from build123d import *

# Parameters (mm, degrees)
SKETCH1_R           = 30
BOSS_EXTRUDE1_DEPTH = 21.25
CUT_EXTRUDE1_DEPTH  = 5
SKETCH5_R           = 1.8
CUT_EXTRUDE2_DEPTH  = 48.45063224
CUT_EXTRUDE3_DEPTH  = 13
SKETCH10_W          = 15
SKETCH10_H          = 9.25
CUT_EXTRUDE6_DEPTH  = 28
FILLET6_R           = 5
FILLET7_R           = 5


with BuildPart() as part:
    # Sketch1 → Boss-Extrude1 (new body)
    with BuildSketch(Plane.XY):
        Circle(SKETCH1_R)
    extrude(amount=BOSS_EXTRUDE1_DEPTH)

    # Sketch2 → Cut-Extrude1 (cut)
    with BuildSketch(Plane.XY.offset(21.25)):
        Polygon((0, 7.361215932), (-6.375, 3.680607966), (-6.375, -3.680607966), (0, -7.361215932), (6.375, -3.680607966), (6.375, 3.680607966), align=None)
    extrude(amount=-CUT_EXTRUDE1_DEPTH, mode=Mode.SUBTRACT)

    # Sketch4 → Cut-Revolve1 (revolve, cut)
    with BuildSketch(Plane(origin=(0, 0, 0), x_dir=(1, 0, 0), z_dir=(0, 1, 0)), mode=Mode.PRIVATE) as cut_revolve1_sk:
        Polygon((30, -19.25), (26, -15.25), (26, -6), (30, -2), align=None)
    revolve(cut_revolve1_sk.sketch.rotate(Axis((0, 0, -12.64061748), (0, 0, 1)), 180), axis=Axis((0, 0, -12.64061748), (0, 0, 1)), mode=Mode.SUBTRACT)

    # Sketch5 → Cut-Extrude2 (cut, through all)
    with BuildSketch(Plane.XY.offset(21.25)):
        with Locations((-17.320508076, -10)):
            Circle(SKETCH5_R)
        with Locations((17.320508076, -10)):
            Circle(SKETCH5_R)
        with Locations((0, 20)):
            Circle(SKETCH5_R)
    extrude(amount=-CUT_EXTRUDE2_DEPTH, mode=Mode.SUBTRACT)

    # Sketch6 → Cut-Extrude3 (cut)
    with BuildSketch(Plane(origin=(0, 0, 0), x_dir=(-1, 0, 0), z_dir=(0, 0, -1))):
        Polygon((7.361215932, 0), (3.680607966, 6.375), (-3.680607966, 6.375), (-7.361215932, 0), (-3.680607966, -6.375), (3.680607966, -6.375), align=None)
    extrude(amount=-CUT_EXTRUDE3_DEPTH, mode=Mode.SUBTRACT)

    # Sketch10 → Cut-Extrude6 (cut)
    with BuildSketch(Plane(origin=(0, 40, 0), x_dir=(1, 0, 0), z_dir=(0, 1, 0))):
        with Locations((0, -10.625)):
            Rectangle(SKETCH10_W, SKETCH10_H)
    extrude(amount=-CUT_EXTRUDE6_DEPTH, mode=Mode.SUBTRACT)

    # Fillet6
    fillet6_edges = [part.edges().sort_by_distance(p)[0] for p in [
        (-7.5, 24.894778569, 10.625),
        (7.5, 24.894778569, 10.625),
    ]]
    fillet(fillet6_edges, radius=FILLET6_R)

    # Fillet7
    fillet7_edges = [part.edges().sort_by_distance(p)[0] for p in [
        (7.5, 12, 10.625),
        (-7.5, 12, 10.625),
    ]]
    fillet(fillet7_edges, radius=FILLET7_R)


solid = part.part
Input: part model. Units: mm. Frame: model coordinates. A direction names the side the tool comes from. Give positions to 0.01 mm unless a question says otherwise; leave off trailing zeros. Order: outer loops, then holes, each group sorted by start corner. A loop starts at its lowest first (then second) coordinate and runs counter-clockwise, first axis right, second up.
Q1. Ray query, probe 1 along X at (y, z) = (-8.5, 13.25); probe 2 along Z at (x, y) = (7, 15); probe 3 along Y at (x, z) = (0, 16.6). Return the intervals inside material, ascending.
Checked values:
probe 1: x = -24.57 to -18.32, -16.33 to 16.33, 18.32 to 24.57
probe 2: z = 0 to 6, 15.25 to 21.25
probe 3: y = -27.35 to -7.36, 7.36 to 18.2, 21.8 to 27.35
Q2. Section B-B on z = 18.25. Output: boundary loops of the cut face in (x, y) (1 decimal), and give its area (3 significant figures).
Checked values:
outline: circle Ø58 at (0, 0); hole circle Ø3.6 at (-17.3, -10); hole (-6.4, -3.7) - (0, -7.4) - (6.4, -3.7) - (6.4, 3.7) - (0, 7.4) - (-6.4, 3.7) - close; hole circle Ø3.6 at (0, 20); hole circle Ø3.6 at (17.3, -10)
area: 2,470 mm2
Q3. Section A-A on z = 3.5. Output: boundary loops of the cut face in (x, y) (1 decimal), and give its area (3 significant figures).
Checked values:
outline: circle Ø57 at (0, 0); hole circle Ø3.6 at (-17.3, -10); hole (-7.4, 0) - (-3.7, -6.4) - (3.7, -6.4) - (7.4, 0) - (3.7, 6.4) - (-3.7, 6.4) - close; hole circle Ø3.6 at (0, 20); hole circle Ø3.6 at (17.3, -10)
area: 2,380 mm2
Q4. Draft query along X for faces 4 (the cylindrical face through (-0.911, -25.984, 10.56)), 5 (the flat face through (0, 12, 11)). Return one class per face: +X half, -X half, draft (parallel to the pull), parting line (faces both ways), or undercut.
Checked values:
face 4: parting line
face 5: undercut
Q5. Set-up query: faces 1 (the flat face through (0, 18, 15.25)), 2 (the flat face through (0, 0, 13)), 3 (the flat face through (-3.14, 5.55, 18.78)). Return all of +Z, -Z, +X, -X, +Y, -Y with unobstructed straight access to the full face (end or side cutting, diameter ignored); none if empty.
Checked values:
face 1: +Y
face 2: -Z
face 3: +Z
Q6. Contact query for flat-ended pins moving along their axis: pin 1 Ø2.5 at (y, z) = (-0.5, 19.5) entering from +X; pin 2 Ø2 at (x, z) = (-1, 6.5) entering from -Y; pin 3 Ø1.5 at (x, z) = (-21, 8.5) entering from +Y; pin 4 Ø2 at (x, y) = (0, 20) entering from -Z. Output: stop coordinate, or through.
Checked values:
pin 1: stops at x = 30
pin 2: stops at y = -26.48
pin 3: stops at y = 16.31
pin 4: passes through
Q7. Section C-C on y = -10. State how many separate pieces and enclosed holes the cut face has, and give its area (3 significant figures).
Checked values:
separate pieces: 3
enclosed holes: 0
area: 936 mm2
